Here's how the part is built. I have some questions about the finished solid (model axes, mm). Give positions to 0.01 mm unless a question says otherwise; leave off trailing zeros. Write each loop counter-clockwise with the first axis right and the second up, starting at its lowest first coordinate (ties: lowest second). Pieces come first, ordered by that corner, then holes. Notation, with made-up numbers: (82, 25.25) -> (128, 25.25) arc R17 ccw to (128, 40.25) -> close; hole circle Ø5 at (64, 83). An arc over 180 degrees is marked (long way). Use one line per item in the form item = value.
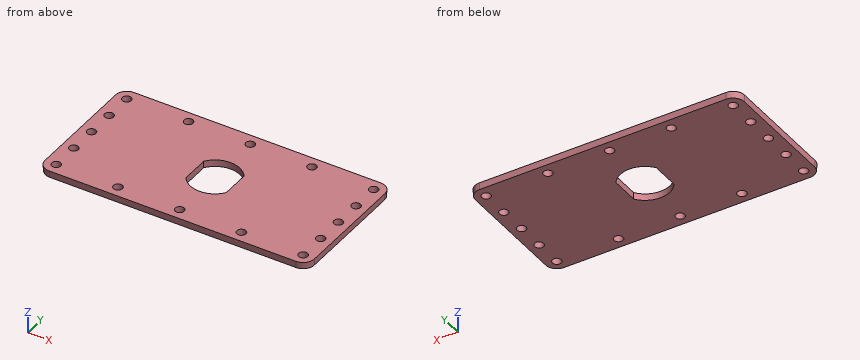
```python
from build123d import *

# Parameters (mm, degrees)
SKETCH1_W           = 120
SKETCH1_H           = 60
BOSS_EXTRUDE1_DEPTH = 3
BOSS_EXTRUDE1_DRAFT = -2.862405226
CUT_EXTRUDE4_DEPTH  = 25
FILLET1_R           = 5
CUT_EXTRUDE5_REACH  = 69.149
SKETCH6_R           = 2


with BuildPart() as part:
    # Sketch1 → Boss-Extrude1 (with draft: the straight prism first)
    with BuildSketch(Plane.XY):
        Rectangle(SKETCH1_W, SKETCH1_H)
    extrude(amount=-BOSS_EXTRUDE1_DEPTH)
    # Boss-Extrude1: the draft: its side faces are tilted about the plane it starts from
    boss_extrude1_sides = [part.faces().sort_by_distance(p)[0] for p in [
        (0, -30, -1.5),
        (60, 0, -1.5),
        (0, 30, -1.5),
        (-60, 0, -1.5),
    ]]
    draft(boss_extrude1_sides, Plane.XY, BOSS_EXTRUDE1_DRAFT)

    # Sketch5 → Cut-Extrude4 (cut)
    with BuildSketch(Plane.XY):
        with BuildLine():
            Line((-9, 6.32455532), (-9, -6.32455532))
            ThreePointArc((-9, -6.32455532), (0, -11), (9, -6.32455532))
            Line((9, -6.32455532), (9, 6.32455532))
            ThreePointArc((9, 6.32455532), (0, 11), (-9, 6.32455532))
        make_face()
    extrude(amount=-CUT_EXTRUDE4_DEPTH, mode=Mode.SUBTRACT)

    # Fillet1
    fillet1_edges = [part.edges().sort_by_distance(p)[0] for p in [
        (59.925, -29.925, -1.5),
        (-59.925, -29.925, -1.5),
        (-59.925, 29.925, -1.5),
        (59.925, 29.925, -1.5),
    ]]
    fillet(fillet1_edges, radius=FILLET1_R)

    # Sketch6 → Cut-Extrude5 (cut, up to next)
    with BuildSketch(Plane.XY, mode=Mode.PRIVATE) as cut_extrude5_sk1:
        with Locations((-55, 25)):
            Circle(SKETCH6_R)
    cut_extrude5_tool1 = extrude(cut_extrude5_sk1.sketch, amount=-CUT_EXTRUDE5_REACH, mode=Mode.PRIVATE) & part.part
    # Sketch6 → Cut-Extrude5 (cut, up to next)
    with BuildSketch(Plane.XY, mode=Mode.PRIVATE) as cut_extrude5_sk2:
        with Locations((-27.5, 25)):
            Circle(SKETCH6_R)
    cut_extrude5_tool2 = extrude(cut_extrude5_sk2.sketch, amount=-CUT_EXTRUDE5_REACH, mode=Mode.PRIVATE) & part.part
    # Sketch6 → Cut-Extrude5 (cut, up to next)
    with BuildSketch(Plane.XY, mode=Mode.PRIVATE) as cut_extrude5_sk3:
        with Locations((0, 25)):
            Circle(SKETCH6_R)
    cut_extrude5_tool3 = extrude(cut_extrude5_sk3.sketch, amount=-CUT_EXTRUDE5_REACH, mode=Mode.PRIVATE) & part.part
    # Sketch6 → Cut-Extrude5 (cut, up to next)
    with BuildSketch(Plane.XY, mode=Mode.PRIVATE) as cut_extrude5_sk4:
        with Locations((27.5, 25)):
            Circle(SKETCH6_R)
    cut_extrude5_tool4 = extrude(cut_extrude5_sk4.sketch, amount=-CUT_EXTRUDE5_REACH, mode=Mode.PRIVATE) & part.part
    # Sketch6 → Cut-Extrude5 (cut, up to next)
    with BuildSketch(Plane.XY, mode=Mode.PRIVATE) as cut_extrude5_sk5:
        with Locations((55, 25)):
            Circle(SKETCH6_R)
    cut_extrude5_tool5 = extrude(cut_extrude5_sk5.sketch, amount=-CUT_EXTRUDE5_REACH, mode=Mode.PRIVATE) & part.part
    # Sketch6 → Cut-Extrude5 (cut, up to next)
    with BuildSketch(Plane.XY, mode=Mode.PRIVATE) as cut_extrude5_sk6:
        with Locations((55, -25)):
            Circle(SKETCH6_R)
    cut_extrude5_tool6 = extrude(cut_extrude5_sk6.sketch, amount=-CUT_EXTRUDE5_REACH, mode=Mode.PRIVATE) & part.part
    # Sketch6 → Cut-Extrude5 (cut, up to next)
    with BuildSketch(Plane.XY, mode=Mode.PRIVATE) as cut_extrude5_sk7:
        with Locations((27.5, -25)):
            Circle(SKETCH6_R)
    cut_extrude5_tool7 = extrude(cut_extrude5_sk7.sketch, amount=-CUT_EXTRUDE5_REACH, mode=Mode.PRIVATE) & part.part
    # Sketch6 → Cut-Extrude5 (cut, up to next)
    with BuildSketch(Plane.XY, mode=Mode.PRIVATE) as cut_extrude5_sk8:
        with Locations((0, -25)):
            Circle(SKETCH6_R)
    cut_extrude5_tool8 = extrude(cut_extrude5_sk8.sketch, amount=-CUT_EXTRUDE5_REACH, mode=Mode.PRIVATE) & part.part
    # Sketch6 → Cut-Extrude5 (cut, up to next)
    with BuildSketch(Plane.XY, mode=Mode.PRIVATE) as cut_extrude5_sk9:
        with Locations((-27.5, -25)):
            Circle(SKETCH6_R)
    cut_extrude5_tool9 = extrude(cut_extrude5_sk9.sketch, amount=-CUT_EXTRUDE5_REACH, mode=Mode.PRIVATE) & part.part
    # Sketch6 → Cut-Extrude5 (cut, up to next)
    with BuildSketch(Plane.XY, mode=Mode.PRIVATE) as cut_extrude5_sk10:
        with Locations((-55, -25)):
            Circle(SKETCH6_R)
    cut_extrude5_tool10 = extrude(cut_extrude5_sk10.sketch, amount=-CUT_EXTRUDE5_REACH, mode=Mode.PRIVATE) & part.part
    # Sketch6 → Cut-Extrude5 (cut, up to next)
    with BuildSketch(Plane.XY, mode=Mode.PRIVATE) as cut_extrude5_sk11:
        with Locations((-55, 12.5)):
            Circle(SKETCH6_R)
    cut_extrude5_tool11 = extrude(cut_extrude5_sk11.sketch, amount=-CUT_EXTRUDE5_REACH, mode=Mode.PRIVATE) & part.part
    # Sketch6 → Cut-Extrude5 (cut, up to next)
    with BuildSketch(Plane.XY, mode=Mode.PRIVATE) as cut_extrude5_sk12:
        with Locations((-55, 0)):
            Circle(SKETCH6_R)
    cut_extrude5_tool12 = extrude(cut_extrude5_sk12.sketch, amount=-CUT_EXTRUDE5_REACH, mode=Mode.PRIVATE) & part.part
    # Sketch6 → Cut-Extrude5 (cut, up to next)
    with BuildSketch(Plane.XY, mode=Mode.PRIVATE) as cut_extrude5_sk13:
        with Locations((-55, -12.5)):
            Circle(SKETCH6_R)
    cut_extrude5_tool13 = extrude(cut_extrude5_sk13.sketch, amount=-CUT_EXTRUDE5_REACH, mode=Mode.PRIVATE) & part.part
    # Sketch6 → Cut-Extrude5 (cut, up to next)
    with BuildSketch(Plane.XY, mode=Mode.PRIVATE) as cut_extrude5_sk14:
        with Locations((55, -12.5)):
            Circle(SKETCH6_R)
    cut_extrude5_tool14 = extrude(cut_extrude5_sk14.sketch, amount=-CUT_EXTRUDE5_REACH, mode=Mode.PRIVATE) & part.part
    # Sketch6 → Cut-Extrude5 (cut, up to next)
    with BuildSketch(Plane.XY, mode=Mode.PRIVATE) as cut_extrude5_sk15:
        with Locations((55, 0)):
            Circle(SKETCH6_R)
    cut_extrude5_tool15 = extrude(cut_extrude5_sk15.sketch, amount=-CUT_EXTRUDE5_REACH, mode=Mode.PRIVATE) & part.part
    # Sketch6 → Cut-Extrude5 (cut, up to next)
    with BuildSketch(Plane.XY, mode=Mode.PRIVATE) as cut_extrude5_sk16:
        with Locations((55, 12.5)):
            Circle(SKETCH6_R)
    cut_extrude5_tool16 = extrude(cut_extrude5_sk16.sketch, amount=-CUT_EXTRUDE5_REACH, mode=Mode.PRIVATE) & part.part
    add(cut_extrude5_tool1.solids().sort_by_distance((-55, 25, 0))[0], mode=Mode.SUBTRACT)
    add(cut_extrude5_tool2.solids().sort_by_distance((-27.5, 25, 0))[0], mode=Mode.SUBTRACT)
    add(cut_extrude5_tool3.solids().sort_by_distance((0, 25, 0))[0], mode=Mode.SUBTRACT)
    add(cut_extrude5_tool4.solids().sort_by_distance((27.5, 25, 0))[0], mode=Mode.SUBTRACT)
    add(cut_extrude5_tool5.solids().sort_by_distance((55, 25, 0))[0], mode=Mode.SUBTRACT)
    add(cut_extrude5_tool6.solids().sort_by_distance((55, -25, 0))[0], mode=Mode.SUBTRACT)
    add(cut_extrude5_tool7.solids().sort_by_distance((27.5, -25, 0))[0], mode=Mode.SUBTRACT)
    add(cut_extrude5_tool8.solids().sort_by_distance((0, -25, 0))[0], mode=Mode.SUBTRACT)
    add(cut_extrude5_tool9.solids().sort_by_distance((-27.5, -25, 0))[0], mode=Mode.SUBTRACT)
    add(cut_extrude5_tool10.solids().sort_by_distance((-55, -25, 0))[0], mode=Mode.SUBTRACT)
    add(cut_extrude5_tool11.solids().sort_by_distance((-55, 12.5, 0))[0], mode=Mode.SUBTRACT)
    add(cut_extrude5_tool12.solids().sort_by_distance((-55, 0, 0))[0], mode=Mode.SUBTRACT)
    add(cut_extrude5_tool13.solids().sort_by_distance((-55, -12.5, 0))[0], mode=Mode.SUBTRACT)
    add(cut_extrude5_tool14.solids().sort_by_distance((55, -12.5, 0))[0], mode=Mode.SUBTRACT)
    add(cut_extrude5_tool15.solids().sort_by_distance((55, 0, 0))[0], mode=Mode.SUBTRACT)
    add(cut_extrude5_tool16.solids().sort_by_distance((55, 12.5, 0))[0], mode=Mode.SUBTRACT)


solid = part.part
```
Q1. Will these pins go through, and if not, where does the flat tip stop? pin 1 Ø3.5 at (x, y) = (-55, -25) entering from -Z; pin 2 Ø1 at (x, z) = (10, -2) entering from -Y (3 decimals); pin 3 Ø1.5 at (y, z) = (1.5, -1.5) entering from -X; pin 4 Ø1 at (y, z) = (-10.5, -2) entering from -X (3 decimals).
Result set:
pin_1 = through
pin_2 = -29.925
pin_3 = -59.96
pin_4 = -59.925
Q2. I want a section at A-A, the plane x = 27.5. Write out the boundary of the cut face in (y, z), and give its area (3 significant figures).
Result set:
outline = (-30, 0) -> (-29.85, -3) -> (-27, -3) -> (-27, 0) -> close; (-23, -3) -> (23, -3) -> (23, 0) -> (-23, 0) -> close; (27, -3) -> (29.85, -3) -> (30, 0) -> (27, 0) -> close
area = 156 mm2
Q3. If I drill on line 1 along Y through (x, z) = (55, -1.75); line 2 along X through (y, z) = (26, -0.25); line 3 along X through (y, z) = (-21.5, -2.75), over which ranges is the centre line in solid material (lowest first)? Write a range as from..to.
Result set:
line_1 = -29.91..-27, -23..-14.5, -10.5..-2, 2..10.5, 14.5..23, 27..29.91
line_2 = -59.89..-56.73, -53.27..-29.23, -25.77..-1.73, 1.73..25.77, 29.23..53.27, 56.73..59.89
line_3 = -59.86..59.86
Q4. I want a section at B-B, the plane y = 12.5. Write out the boundary of the cut face in (x, z), and give its area (3 significant figures).
Result set:
outline = (-60, 0) -> (-59.85, -3) -> (-57, -3) -> (-57, 0) -> close; (-53, -3) -> (53, -3) -> (53, 0) -> (-53, 0) -> close; (57, -3) -> (59.85, -3) -> (60, 0) -> (57, 0) -> close
area = 336 mm2
Q5. I want a section at C-C, the plane z = -1.35. Count the separate pieces of the cut face and the enclosed holes in it, and give its area (3 significant figures).
Result set:
separate_pieces = 1
enclosed_holes = 17
area = 6,610 mm2
